Here's how the part is built. I have some questions about the finished solid (model axes, mm). A direction names the side the tool comes from. Round coordinates to 2 decimals unless told otherwise and drop trailing zeros. Order: outer loops, then holes, each group sorted by start corner. A loop starts at its lowest first (then second) coordinate and runs counter-clockwise, first axis right, second up. Notation, with made-up numbers: (13.5, 42.25) -> (17.5, 42.25) arc R7 cw to (17.5, 52.25) -> close; hole circle Ø2 at (27.5, -19.5). An arc over 180 degrees is marked (long way). Use a Markdown table: item, result. Add a question column.
(1) I want a section at C-C, the plane y = 0.75. Please give me the cut outline in (x, z), then the cut area to 3 significant figures.
(2) Thinking about a two-plate mould opening in X: for faces 3 (the face through (-10.74, 0.07, -2.38)), 4 (the face through (2, -6, -9)), 5 (the face through (2.703, 5.493, 8.584)), which applies, pulls with the +X half, pulls with the -X half, needs draft (parallel to the pull), parting line crosses it, or undercut?
(3) I want a section at B-B, the plane z = 0. Please give me the cut outline in (x, y), then the cut area to 3 significant figures.
(4) I'm going to push flat-ended pins straight in: P1, Ø9, axis at x = -1, z = -4, coming from the -Y side; P2, Ø9, axis at x = 2.5, z = -1.5, coming from the +Y side; P3, Ø3, axis at y = 2, z = 5, coming from the +X side. Where does each tip first touch, or does it pass through?
(5) If I drill on probe 1 along Y at (x, z) = (2.5, -8.5); probe 2 along X at (y, z) = (-0.25, 0); probe 3 along Z at (x, y) = (4.5, -4), over which ranges is the centre line in solid material (lowest first)?
(6) On a 3-axis mill with a long thin cutter (end or side, diameter ignored), from which of +Z, -Z, +X, -X, +Y, -Y can I reach the whole of each face in a straight line? I mean faces 1 (the face through (-7.81, -0.07, -1.73)), 2 (the face through (2.703, -5.493, 8.584)). Say none if no direction works.
(7) I want a section at A-A, the plane x = 0. Please give me the cut outline in (y, z).
from build123d import *

# Parameters (mm, degrees)
SKETCH1_R           = 11
SKETCH1_R_2         = 8
BOSS_EXTRUDE1_DEPTH = 6
FILLET1_R           = 1
CUT_EXTRUDE1_START  = -1
SKETCH2_R           = 9
SKETCH2_R_2         = 8
CUT_EXTRUDE1_DEPTH  = 1


with BuildPart() as part:
    # Sketch1 → Boss-Extrude1 (new, symmetric)
    with BuildSketch(Plane(origin=(0, 0, 0), x_dir=(1, 0, 0), z_dir=(0, 1, 0))):
        with Locations(Location((0, 0, 0), (0, 0, 270))):
            Circle(SKETCH1_R)
        with Locations(Location((0, 0, 0), (0, 0, 270))):
            Circle(SKETCH1_R_2, mode=Mode.SUBTRACT)
    extrude(amount=BOSS_EXTRUDE1_DEPTH, both=True)

    # Fillet1
    fillet1_edges = [part.edges().sort_by_distance(p)[0] for p in [
        (0, -6, -11),
        (0, 6, -11),
    ]]
    fillet(fillet1_edges, radius=FILLET1_R)

    # Sketch2 → Cut-Extrude1 (cut)
    with BuildSketch(Plane(origin=(0, 6, 0), x_dir=(1, 0, 0), z_dir=(0, 1, 0)).offset(CUT_EXTRUDE1_START)):
        with Locations(Location((0, 0, 0), (0, 0, 270))):
            Circle(SKETCH2_R)
        with Locations(Location((0, 0, 0), (0, 0, 270))):
            Circle(SKETCH2_R_2, mode=Mode.SUBTRACT)
    cut_extrude1 = extrude(amount=CUT_EXTRUDE1_DEPTH, mode=Mode.SUBTRACT)

    # Mirror1: Cut-Extrude1 across plane
    add(cut_extrude1.mirror(Plane.ZX), mode=Mode.SUBTRACT)


solid = part.part
Taken from the geometry:
| question | item | result |
|---|---|---|
| 1 | outline | circle Ø22 at (0, 0); hole circle Ø16 at (0, 0) |
| 1 | area | 179 mm2 |
| 2 | face 3 | parting line crosses it |
| 2 | face 4 | needs draft |
| 2 | face 5 | undercut |
| 3 | outline | (-11, -5) arc R1 ccw to (-10, -6) -> (-9, -6) -> (-9, -5) -> (-8, -5) -> (-8, 5) -> (-9, 5) -> (-9, 6) -> (-10, 6) arc R1 ccw to (-11, 5) -> close; (8, -5) -> (9, -5) -> (9, -6) -> (10, -6) arc R1 ccw to (11, -5) -> (11, 5) arc R1 ccw to (10, 6) -> (9, 6) -> (9, 5) -> (8, 5) -> close |
| 3 | area | 67.1 mm2 |
| 4 | P1 | stops at y = -5 |
| 4 | P2 | passes through |
| 4 | P3 | stops at x = 10.43 |
| 5 | probe 1 | y = -5 to 5 |
| 5 | probe 2 | x = -11 to -8, 8 to 11 |
| 5 | probe 3 | z = -10.04 to -6.61, 6.61 to 10.04 |
| 6 | face 1 | +Y, -Y |
| 6 | face 2 | -Y |
| 7 | outline | (-6, -10) arc R1 ccw to (-5, -11) -> (5, -11) arc R1 ccw to (6, -10) -> (6, -9) -> (5, -9) -> (5, -8) -> (-5, -8) -> (-5, -9) -> (-6, -9) -> close; (-6, 9) -> (-5, 9) -> (-5, 8) -> (5, 8) -> (5, 9) -> (6, 9) -> (6, 10) arc R1 ccw to (5, 11) -> (-5, 11) arc R1 ccw to (-6, 10) -> close |
